Geometry check sheet. Reference: the model listing, model coordinates, mm. Face numbers are marked on the shaded views. A direction names the side the tool comes from. Round coordinates to 2 decimals unless told otherwise and drop trailing zeros. Order: outer loops, then holes, each group sorted by start corner. A loop starts at its lowest first (then second) coordinate and runs counter-clockwise, first axis right, second up. Notation, with made-up numbers: (21.5, 15) - (40.5, 15) arc R20 cw to (40.5, 21) - close; hole circle Ø2 at (-16, -9). An arc over 180 degrees is marked (long way). Use a Markdown table: item, result. Add a question column.
(1) Access from +Z, -Z, +X, -X, +Y, -Y to the whole of each face (thin tool, end or side, straight path). Record for the marked faces 3, 4 and 5.
(2) Section check B-B on z = -19.5. Record the boundary of the cut face in (x, y), then the cut area to 3 significant figures.
(3) Section check C-C on x = 26.5. Record the boundary of the cut face in (y, z), then the cut area to 3 significant figures.
(4) Thickness scan on line 1 along Z through (x, y) = (-52.07, 1.3); line 2 along Y through (x, z) = (-49, 0). Record the ranges inside material, lowest first. Write a range as [from, to].
(5) Mould release check, pull along X, two halves, no side actions. Record for the marked faces 1 and 2: released by +X, released by -X, zero draft, split by the parting line, or undercut.
(6) Section check A-A on x = 50.5. Record the boundary of the cut face in (y, z).
(7) Gauge pin test, flat ends, axial feed: P1, Ø6, axis at x = -52.07, z = -28.575, coming from the +Y side; P2, Ø4, axis at y = -3, z = 45, coming from the -X side; P3, Ø1.5, axis at y = -13, z = 5.5, coming from the +X side; P4, Ø9, axis at x = 1.5, y = -9, coming from the -Z side. Record the tip position at first contact, or that the pin passes through.
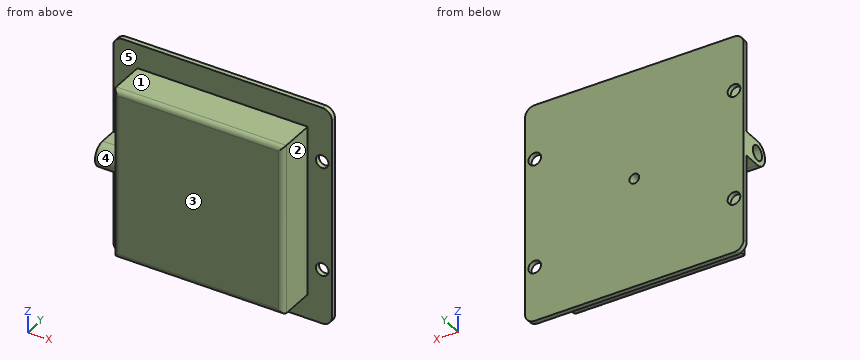
```python
from build123d import *

# Parameters (mm, degrees)
SKETCH1_W                   = 114.3
SKETCH1_H                   = 114.3
BOSS_EXTRUDE1_DEPTH         = 2.54
SKETCH2_W                   = 88.9
SKETCH2_H                   = 88.9
BOSS_EXTRUDE2_DEPTH         = 20.32
G_0_261_DIAMETER_HOLE1_D    = 6.6294
FILLET1_R                   = 2.54
FILLET2_R                   = 5.08
BOSS_EXTRUDE3_DEPTH         = 12.7
SKETCH8_R                   = 3.81
CUT_EXTRUDE1_DEPTH          = 12.7
F_1_4_20_TAPPED_HOLE1_D     = 5.1054
F_1_4_20_TAPPED_HOLE1_DEPTH = 16.51
F_1_4_20_TAPPED_HOLE1_TIP   = 1.533816902


with BuildPart() as part:
    # Sketch1 → Boss-Extrude1 (new body)
    with BuildSketch(Plane(origin=(0, 0, 0), x_dir=(1, 0, 0), z_dir=(0, 1, 0))):
        Rectangle(SKETCH1_W, SKETCH1_H)
    extrude(amount=BOSS_EXTRUDE1_DEPTH)

    # Sketch2 → Boss-Extrude2 (add)
    with BuildSketch(Plane.XZ):
        Rectangle(SKETCH2_W, SKETCH2_H)
    extrude(amount=BOSS_EXTRUDE2_DEPTH)

    # G (0.261) Diameter Hole1 (through all)
    with Locations(Plane(origin=(0, 0, 0), x_dir=(-1, 0, 0), z_dir=(0, -1, 0))):
        with Locations((52.07, -28.575), (52.07, 28.575), (-52.07, -28.575), (-52.07, 28.575)):
            Hole(G_0_261_DIAMETER_HOLE1_D / 2)

    # Fillet1
    fillet1_edges = [part.edges().sort_by_distance(p)[0] for p in [
        (44.45, -20.32, 0),
        (0, -20.32, 44.45),
        (-44.45, -20.32, 0),
        (0, -20.32, -44.45),
    ]]
    fillet(fillet1_edges, radius=FILLET1_R)

    # Fillet2
    fillet2_edges = [part.edges().sort_by_distance(p)[0] for p in [
        (-57.15, 1.27, -57.15),
        (57.15, 1.27, -57.15),
        (57.15, 1.27, 57.15),
        (-57.15, 1.27, 57.15),
    ]]
    fillet(fillet2_edges, radius=FILLET2_R)

    # Sketch5 → Boss-Extrude3 (add)
    with BuildSketch(Plane.ZY.offset(44.45)):
        with BuildLine():
            ThreePointArc((-6.35, -8.89), (0, -15.24), (6.35, -8.89))
            Line((6.35, -8.89), (-6.35, -8.89))
        make_face()
        with BuildLine():
            Line((-6.35, -8.89), (6.35, -8.89))
            ThreePointArc((6.35, -8.89), (0, -2.54), (-6.35, -8.89))
        make_face()
        with BuildLine():
            ThreePointArc((-6.35, -8.89), (0, -2.54), (6.35, -8.89))
            Line((6.35, -8.89), (6.35, 0))
            Line((6.35, 0), (-6.35, 0))
            Line((-6.35, 0), (-6.35, -8.89))
        make_face()
    extrude(amount=BOSS_EXTRUDE3_DEPTH)

    # Sketch8 → Cut-Extrude1 (cut)
    with BuildSketch(Plane.ZY.offset(57.15)):
        with Locations((0, -8.89)):
            Circle(SKETCH8_R)
    extrude(amount=-CUT_EXTRUDE1_DEPTH, mode=Mode.SUBTRACT)

    # 1/4-20 Tapped Hole1
    with Locations(Plane(origin=(0, 2.54, 0), x_dir=(1, 0, 0), z_dir=(0, 1, 0))):
        with Locations((0, 0)):
            Hole(F_1_4_20_TAPPED_HOLE1_D / 2, depth=F_1_4_20_TAPPED_HOLE1_DEPTH)
            with Locations((0, 0, -(F_1_4_20_TAPPED_HOLE1_DEPTH + F_1_4_20_TAPPED_HOLE1_TIP / 2))):  # 118° drill point
                Cone(0, F_1_4_20_TAPPED_HOLE1_D / 2, F_1_4_20_TAPPED_HOLE1_TIP, mode=Mode.SUBTRACT)


solid = part.part
```
Check sheet entries:
| question | item | result |
|---|---|---|
| 1 | face 3 | +Z, -Z, +X, -X, -Y |
| 1 | face 4 | -X, -Y |
| 1 | face 5 | -Y |
| 2 | outline | (-57.15, 0) - (-44.45, 0) - (-44.45, -17.78) arc R2.54 ccw to (-41.91, -20.32) - (41.91, -20.32) arc R2.54 ccw to (44.45, -17.78) - (44.45, 0) - (57.15, 0) - (57.15, 2.54) - (-57.15, 2.54) - close |
| 2 | area | 2,090 mm2 |
| 3 | outline | (-20.32, -41.91) arc R2.54 ccw to (-17.78, -44.45) - (0, -44.45) - (0, -57.15) - (2.54, -57.15) - (2.54, 57.15) - (0, 57.15) - (0, 44.45) - (-17.78, 44.45) arc R2.54 ccw to (-20.32, 41.91) - close |
| 3 | area | 2,090 mm2 |
| 4 | line 1 | z = [-57.15, -31.89], [-25.26, 25.26], [31.89, 57.15] |
| 4 | line 2 | y = [-15.24, -12.7], [-5.08, 2.54] |
| 5 | face 1 | zero draft |
| 5 | face 2 | released by +X |
| 6 | outline | (0, -57.15) - (2.54, -57.15) - (2.54, -31.49) - (0, -31.49) - close; (0, -25.66) - (2.54, -25.66) - (2.54, 25.66) - (0, 25.66) - close; (0, 31.49) - (2.54, 31.49) - (2.54, 57.15) - (0, 57.15) - close |
| 7 | P1 | passes through |
| 7 | P2 | stops at x = -44.45 |
| 7 | P3 | stops at x = 44.45 |
| 7 | P4 | stops at z = -44.45 |
